Verification items for the finished model (mm, model axes). A direction names the side the tool comes from. Give positions to 0.01 mm unless a question says otherwise; leave off trailing zeros. Loops run counter-clockwise (first coordinate to the right, second up) from the corner with the lowest first, then second, coordinate; pieces in that order, holes last. Notation, with made-up numbers: M -29.75,80 L -3.75,80 A18 cw -3.75,106 Z; hole C -24.75,-3.5 d6. An arc over 180 degrees is marked long. Answer in a Markdown table with one row per item.
```python
from build123d import *

# Parameters (mm, degrees)
SKETCH1_W           = 50
SKETCH1_H           = 45
BOSS_EXTRUDE1_DEPTH = 4
SKETCH2_W           = 38
SKETCH2_H           = 45.007332522
BOSS_EXTRUDE2_DEPTH = 5
SKETCH3_W           = 50
SKETCH3_H           = 38
BOSS_EXTRUDE3_DEPTH = 3
SKETCH4_W           = 38
SKETCH4_H           = 48.007332522
BOSS_EXTRUDE4_DEPTH = 5
SKETCH5_W           = 38
SKETCH5_H           = 29.964277952
CUT_EXTRUDE3_DEPTH  = 4
SKETCH7_R           = 0.75
CUT_EXTRUDE4_DEPTH  = 54


with BuildPart() as part:
    # Sketch1 → Boss-Extrude1 (new body)
    with BuildSketch(Plane.XY):
        Rectangle(SKETCH1_W, SKETCH1_H)
    extrude(amount=BOSS_EXTRUDE1_DEPTH)

    # Sketch2 → Boss-Extrude2 (add)
    with BuildSketch(Plane(origin=(25, 0, 0), x_dir=(0, 0, -1), z_dir=(1, 0, 0))):
        with Locations((15, -0.003666261)):
            Rectangle(SKETCH2_W, SKETCH2_H)
    extrude(amount=-BOSS_EXTRUDE2_DEPTH)

    # Sketch3 → Boss-Extrude3 (add)
    with BuildSketch(Plane(origin=(0, 22.5, 0), x_dir=(1, 0, 0), z_dir=(0, 1, 0))):
        with Locations((0, 15)):
            Rectangle(SKETCH3_W, SKETCH3_H)
    extrude(amount=BOSS_EXTRUDE3_DEPTH)

    # Sketch4 → Boss-Extrude4 (add)
    with BuildSketch(Plane.ZY.offset(25)):
        with Locations((-15, 1.496333739)):
            Rectangle(SKETCH4_W, SKETCH4_H)
    extrude(amount=-BOSS_EXTRUDE4_DEPTH)

    # Sketch5 → Cut-Extrude3 (cut)
    with BuildSketch(Plane(origin=(25, 0, 0), x_dir=(0, 0, -1), z_dir=(1, 0, 0))):
        with Locations((15, 0)):
            Rectangle(SKETCH5_W, SKETCH5_H)
    extrude(amount=-CUT_EXTRUDE3_DEPTH, mode=Mode.SUBTRACT)

    # Sketch7 → Cut-Extrude4 (cut)
    with BuildSketch(Plane.ZY.offset(25)):
        with Locations(Location((-15, 0, 0), (0, 0, 90))):
            Circle(SKETCH7_R)
    extrude(amount=-CUT_EXTRUDE4_DEPTH, mode=Mode.SUBTRACT)


solid = part.part
```
Item 1: Sectioned sample at D-D (x = -17). Record the cut outline in (y, z), and give its area (3 significant figures).
Reported:
| item | result |
|---|---|
| outline | M -22.5,0 L 22.5,0 L 22.5,-34 L 25.5,-34 L 25.5,4 L -22.5,4 Z |
| area | 294 mm^2 |
Item 2: Sectioned sample at C-C (z = -15). Record the cut outline in (x, y), and give its area (3 significant figures).
Reported:
| item | result |
|---|---|
| outline | M -25,-22.51 L -20,-22.51 L -20,-0.75 L -25,-0.75 Z; M -25,0.75 L -20,0.75 L -20,22.5 L 20,22.5 L 20,0.75 L 21,0.75 L 21,14.98 L 25,14.98 L 25,25.5 L -25,25.5 Z; M 20,-22.51 L 25,-22.51 L 25,-14.98 L 21,-14.98 L 21,-0.75 L 20,-0.75 Z |
| area | 471 mm^2 |
Item 3: Tool access check on faces 4 (the flat face through (23, -14.982, -15)), 5 (the flat face through (20, 0, -19)), 6 (the cylindrical face through (-22.535, 0.403, -15.632)). Record the directions out of +Z, -Z, +X, -X, +Y, -Y that give a thin tool (end or side, any length) a straight path to the whole face; none if there is none.
Reported:
| item | result |
|---|---|
| face 4 | +Z, -Z, +X |
| face 5 | -Z, -Y |
| face 6 | +X, -X |
Item 4: Go/stop test with flat-tipped pins: pin 1 (1.4 mm diameter, centred on y = 0, z = -15, fed in from +X); pin 2 (1 mm diameter, centred on x = -1, y = 2.5, fed in from -Z); pin 3 (17 mm diameter, centred on x = 8.5, z = -15, fed in from -Y); pin 4 (3 mm diameter, centred on x = 0, z = 2, fed in from -Y). Record where each tip stops, or that it passes through.
Reported:
| item | result |
|---|---|
| pin 1 | passes through |
| pin 2 | stops at z = 0 |
| pin 3 | stops at y = 22.5 |
| pin 4 | stops at y = -22.5 |
Item 5: Sectioned sample at B-B (z = -6). Record the cut outline in (x, y).
Reported:
| item | result |
|---|---|
| outline | M -25,-22.51 L -20,-22.51 L -20,22.5 L 20,22.5 L 20,-22.51 L 25,-22.51 L 25,-14.98 L 21,-14.98 L 21,14.98 L 25,14.98 L 25,25.5 L -25,25.5 Z |
Item 6: Sectioned sample at A-A (y = 0). Record the cut outline in (x, z), and give its area (3 significant figures).
Reported:
| item | result |
|---|---|
| outline | M -25,-34 L -20,-34 L -20,-15.75 L -25,-15.75 Z; M -25,-14.25 L -20,-14.25 L -20,0 L 20,0 L 20,-14.25 L 21,-14.25 L 21,4 L -25,4 Z; M 20,-34 L 21,-34 L 21,-15.75 L 20,-15.75 Z |
| area | 379 mm^2 |
Item 7: Release check for a two-part mould opening along X. For faces 1 (the flat face through (25, 20, -15)), 2 (the flat face through (-4, 23, -34)), 3 (the flat face through (0, 0, 0)) record: released by +X, released by -X, zero draft, split by the parting line, or undercut.
Reported:
| item | result |
|---|---|
| face 1 | released by +X |
| face 2 | zero draft |
| face 3 | undercut |
Item 8: Scan lines: L1, parallel to Y at x = -21.5, z = -15; L2, parallel to X at y = 22, z = -1.5; L3, parallel to X at y = 11.5, z = -8.5. Record each from-to range of solid material in increasing order. Write a range as [from, to].
Reported:
| item | result |
|---|---|
| L1 | y = [-22.51, -0.75], [0.75, 25.5] |
| L2 | x = [-25, -20], [20, 25] |
| L3 | x = [-25, -20], [20, 21] |
